Geometry: final body of the model. Coordinates: model frame, mm. Face numbers are marked on the shaded views. A direction names the side the tool comes from. Coordinates: 2 decimals unless noted, no trailing zeros. Write each loop counter-clockwise with the first axis right and the second up, starting at its lowest first coordinate (ties: lowest second). Pieces come first, ordered by that corner, then holes.
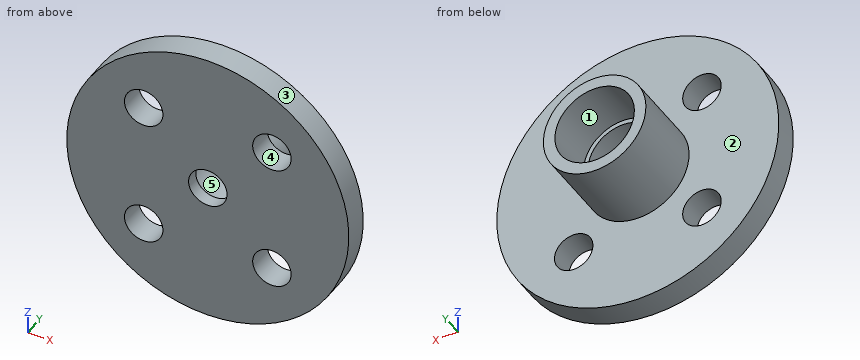
from build123d import *

# Parameters (mm, degrees)
SKETCH_1_R          = 11
SKETCH_1_R_2        = 1.5
EXTRUDE_4_DEPTH     = 2
SKETCH_2_R          = 4
EXTRUDE_5_DEPTH     = 6
SKETCH_3_R          = 3.1
CUT_EXTRUDE_1_DEPTH = 4
SKETCH_4_R          = 2.75
CUT_EXTRUDE_2_DEPTH = 3


with BuildPart() as part:
    # 草图1 → 凸台-拉伸4 (new body)
    with BuildSketch(Plane(origin=(0, 0, 0), x_dir=(1, 0, 0), z_dir=(0, 1, 0))):
        with Locations(Location((0, 0, 0), (0, 0, 270))):
            Circle(SKETCH_1_R)
        with Locations(Location((0, 0, 0), (0, 0, 270))):
            Circle(SKETCH_1_R_2, mode=Mode.SUBTRACT)
        with Locations(Location((-5, 5, 0), (0, 0, 270))):
            Circle(SKETCH_1_R_2, mode=Mode.SUBTRACT)
        with Locations(Location((5, 5, 0), (0, 0, 270))):
            Circle(SKETCH_1_R_2, mode=Mode.SUBTRACT)
        with Locations(Location((5, -5, 0), (0, 0, 270))):
            Circle(SKETCH_1_R_2, mode=Mode.SUBTRACT)
        with Locations(Location((-5, -5, 0), (0, 0, 270))):
            Circle(SKETCH_1_R_2, mode=Mode.SUBTRACT)
    extrude(amount=EXTRUDE_4_DEPTH)

    # 草图2 → 凸台-拉伸5 (add)
    with BuildSketch(Plane(origin=(0, 2, 0), x_dir=(1, 0, 0), z_dir=(0, 1, 0))):
        with Locations(Location((0, 0, 0), (0, 0, 270))):
            Circle(SKETCH_2_R)
    extrude(amount=EXTRUDE_5_DEPTH)

    # 草图3 → 切除-拉伸1 (cut)
    with BuildSketch(Plane(origin=(0, 8, 0), x_dir=(1, 0, 0), z_dir=(0, 1, 0))):
        with Locations(Location((0, 0, 0), (0, 0, 270))):
            Circle(SKETCH_3_R)
    extrude(amount=-CUT_EXTRUDE_1_DEPTH, mode=Mode.SUBTRACT)

    # 草图4 → 切除-拉伸2 (cut)
    with BuildSketch(Plane(origin=(0, 4, 0), x_dir=(1, 0, 0), z_dir=(0, 1, 0))):
        with Locations(Location((0, 0, 0), (0, 0, 270))):
            Circle(SKETCH_4_R)
    extrude(amount=-CUT_EXTRUDE_2_DEPTH, mode=Mode.SUBTRACT)


solid = part.part
Item 1: Material intervals for probe 1 along X at (y, z) = (0.3, 0); probe 2 along X at (y, z) = (2.7, 0); probe 3 along X at (y, z) = (1.5, 5), sorted ascending.
Derived:
probe 1: x = -11 to -1.5, 1.5 to 11
probe 2: x = -4 to -2.75, 2.75 to 4
probe 3: x = -9.8 to -6.5, -3.5 to 3.5, 6.5 to 9.8
Item 2: Pin query (flat end, axial travel): pin 1 (1.6 mm diameter, centred on x = 0.5, z = -1, fed in from +Y); pin 2 (2.5 mm diameter, centred on x = 0, z = 0, fed in from -Y). Return the tip coordinate at first contact, or that it passes through.
Derived:
pin 1: stops at y = 1
pin 2: passes through
Item 3: Section A-A, the plane z = 0. Output: boundary loops of the cut face in (x, y), plus the area to 3 significant figures.
Derived:
outline: (-11, 0) - (-1.5, 0) - (-1.5, 1) - (-2.75, 1) - (-2.75, 4) - (-3.1, 4) - (-3.1, 8) - (-4, 8) - (-4, 2) - (-11, 2) - close; (1.5, 0) - (11, 0) - (11, 2) - (4, 2) - (4, 8) - (3.1, 8) - (3.1, 4) - (2.75, 4) - (2.75, 1) - (1.5, 1) - close
area: 47.7 mm2
Item 4: Section B-B, the plane x = 0. Output: boundary loops of the cut face in (y, z), plus the area to 3 significant figures.
Derived:
outline: (0, -11) - (2, -11) - (2, -4) - (8, -4) - (8, -3.1) - (4, -3.1) - (4, -2.75) - (1, -2.75) - (1, -1.5) - (0, -1.5) - close; (0, 1.5) - (1, 1.5) - (1, 2.75) - (4, 2.75) - (4, 3.1) - (8, 3.1) - (8, 4) - (2, 4) - (2, 11) - (0, 11) - close
area: 47.7 mm2
Item 5: Set-up query: the marked faces 4 and 5. Return all of +Z, -Z, +X, -X, +Y, -Y with unobstructed straight access to the full face (end or side cutting, diameter ignored); none if empty.
Derived:
face 4: +Y, -Y
face 5: +Y
Item 6: Section D-D, the plane y = 7. Output: boundary loops of the cut face in (x, z).
Derived:
outline: circle Ø8 at (0, 0); hole circle Ø6.2 at (0, 0)
Item 7: Pull-direction query (X, two-part tool) for the marked faces 1, 2 and 3; classes: released by +X, released by -X, zero draft, split by the parting line, or undercut.
Derived:
face 1: undercut
face 2: zero draft
face 3: split by the parting line
Item 8: Section C-C, the plane x = -5. Output: boundary loops of the cut face in (y, z), plus the area to 3 significant figures.
Derived:
outline: (0, -9.8) - (2, -9.8) - (2, -6.5) - (0, -6.5) - close; (0, -3.5) - (2, -3.5) - (2, 3.5) - (0, 3.5) - close; (0, 6.5) - (2, 6.5) - (2, 9.8) - (0, 9.8) - close
area: 27.2 mm2
